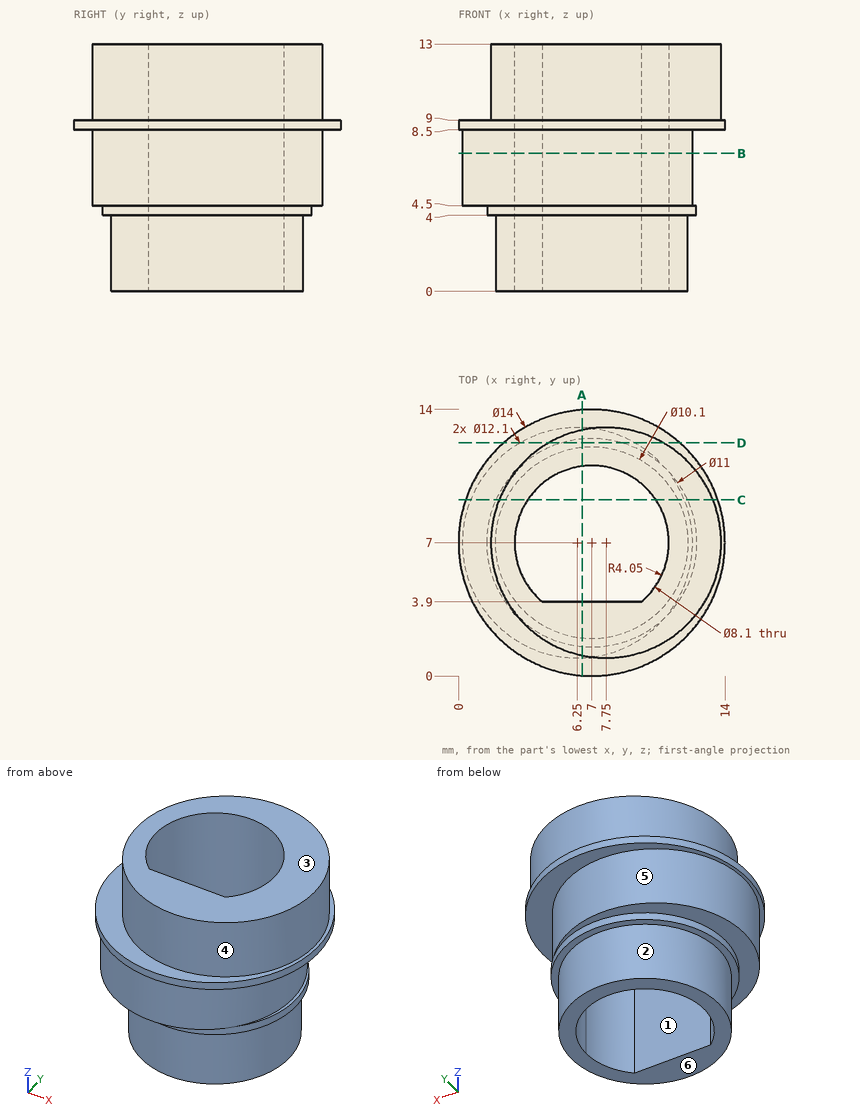
Here's the drawing with two shaded views (mm, measured from the low corner). I have some questions. A direction names the side the tool comes from. Coordinates: 2 decimals unless noted, no trailing zeros. Loops run counter-clockwise (first coordinate to the right, second up) from the corner with the lowest first, then second, coordinate; pieces in that order, holes last. Notation, with made-up numbers: (17.5, 23.5) - (25.5, 23.5) arc R32 cw to (25.5, 62.5) - close; hole circle Ø2 at (-21, 27.25). An arc over 180 degrees is marked (long way). Answer as CSV lines item,"result". Start each with the question number.
1) Suppose I cut it at B-B (z = 7.25). Please give me the cut outline in (x, y).
2) For pin 1 (1 mm diameter, centred on x = 10, z = 10.5, fed in from -Y); pin 2 (6 mm diameter, centred on x = 10.5, z = 8, fed in from +Y), each with a flat end and sliding along its axis, tell me the tip position at first contact or that it passes through.
3) I need wall thicknesses on line 1 (X direction, y = 7, z = 7.25); line 2 (Y direction, x = 7, z = 2.5); line 3 (X direction, y = 8, z = 7.25). Which ranges of each line are inside material? Lowest first, please. Write a range as from..to.
4) Suppose I cut it at A-A (x = 6.5). Please give me the cut outline in (y, z), plus the area to 3 significant figures.
5) Suppose I cut it at D-D (y = 12.25). Please give me the cut outline in (x, z), plus the area to 3 significant figures.
6) Suppose I cut it at C-C (y = 9.25). Please give me the cut outline in (x, z), plus the area to 3 significant figures.
7) Which directions (+Z, -Z, +X, -X, +Y, -Y) give clear straight access to the entire face, cutting with the end or side of a thin tool? Please do the marked faces 4, 5 and 6.
8) Thinking about a two-plate mould opening in Y: for the marked faces 1, 2 and 3, which applies, pulls with the +Y half, pulls with the -Y half, needs draft (parallel to the pull), parting line crosses it, or undercut?
Check result:
1,outline,"circle Ø12.1 at (6.25, 7); hole (4.39, 3.9) - (9.61, 3.9) arc R4.05 ccw (long way) to start"
2,pin 1,"stops at y = 1.21"
2,pin 2,"stops at y = 13.98"
3,line 1,"x = 0.2..2.95, 11.05..12.3"
3,line 2,"y = 1.95..3.9, 11.05..12.05"
3,line 3,"x = 0.28..3.08, 10.92..12.22"
4,outline,"(0.02, 8.5) - (0.96, 8.5) - (0.96, 4.5) - (1.52, 4.5) - (1.52, 4) - (1.97, 4) - (1.97, 0) - (3.9, 0) - (3.9, 13) - (1.08, 13) - (1.08, 9) - (0.02, 9) - close; (11.02, 0) - (12.03, 0) - (12.03, 4) - (12.48, 4) - (12.48, 4.5) - (13.04, 4.5) - (13.04, 8.5) - (13.98, 8.5) - (13.98, 9) - (12.92, 9) - (12.92, 13) - (11.02, 13) - close"
4,area,"55.8 mm²"
5,outline,"(2.37, 8.5) - (3.24, 8.5) - (3.24, 4.5) - (5.36, 4.5) - (5.36, 4) - (8.64, 4) - (8.64, 4.5) - (9.26, 4.5) - (9.26, 8.5) - (11.63, 8.5) - (11.63, 9) - (10.76, 9) - (10.76, 13) - (4.74, 13) - (4.74, 9) - (2.37, 9) - close"
5,area,"54.4 mm²"
6,outline,"(0.37, 8.5) - (0.63, 8.5) - (0.63, 4.5) - (1.98, 4.5) - (1.98, 4) - (2.48, 4) - (2.48, 0) - (3.63, 0) - (3.63, 13) - (2.13, 13) - (2.13, 9) - (0.37, 9) - close; (10.37, 0) - (11.52, 0) - (11.52, 4) - (12.02, 4) - (12.02, 4.5) - (11.87, 4.5) - (11.87, 8.5) - (13.63, 8.5) - (13.63, 9) - (13.37, 9) - (13.37, 13) - (10.37, 13) - close"
6,area,"50.1 mm²"
7,face 4,"+Z"
7,face 5,"none"
7,face 6,"-Z, +X, -X, +Y, -Y"
8,face 1,"undercut"
8,face 2,"parting line crosses it"
8,face 3,"needs draft"
